Input: part model. Units: mm. Frame: model coordinates. A direction names the side the tool comes from. Give positions to 0.01 mm unless a question says otherwise; leave off trailing zeros. Loops run counter-clockwise (first coordinate to the right, second up) from the corner with the lowest first, then second, coordinate; pieces in that order, holes last. Notation, with made-up numbers: M -13,-38 L 15,-38 A17 cw 15,-32 Z; hole C 46,10.25 d7. An arc over 180 degrees is marked long. Answer as a JSON object with one key per item and string values. Group by question number.
1) Access query for faces 1 (the cylindrical face through (-2, 12.6, 0)), 2 (the cylindrical face through (-4, 7.7, -0.1)). Directions: +Z, -Z, +X, -X, +Y, -Y. A direction counts if a zero-diameter tool reaches every point of the face in a straight line with its end or side. Return the directions, or none.
2) Section query A-A on x = 2.5. Return loops of the section in (y, z).
3) First-contact query: P1, Ø8, axis at y = 4.5, z = 6, coming from the +X side; P2, Ø0.6, axis at x = 1, z = -6.5, coming from the +Y side; P3, Ø10, axis at x = -4, z = -3.5, coming from the -Y side. Flat tips, straight axial feed; report the tip coordinate or a pass-through.
4) Section query D-D on z = 8.75. Return loops of the section in (x, y).
5) Section query B-B on y = 6.5. Return loops of the section in (x, z), plus the area to 3 significant figures.
6) Ray query, L1, parallel to X at y = 5.75, z = 7.5; L2, parallel to Y at x = -1, z = 3.5; L3, parallel to Y at x = 0.5, z = 4. Return the intervals inside material, ascending.
7) Section query C-C on z = -1. Return loops of the section in (x, y), plus the area to 3 significant figures.
from build123d import *

# Parameters (mm, degrees)
F2_DEPTH      = 25.4
F2_DEPTH_BACK = 25.4
F3_DEPTH      = 25.4
F3_DEPTH_BACK = 25.4


with BuildPart() as f1:
    # F0 (on Top) → F1 (revolve)
    with BuildSketch(Plane.XY):
        with BuildLine():
            ThreePointArc((1.4741766444, 15.6340406001), (1.7521250826, 17.6942663006), (0, 18.8131241852))
            Line((0, 18.8131241852), (0, 18.009214877))
            ThreePointArc((0, 18.009214877), (0.7972124014, 17.6789986882), (1.1274285902, 16.8817862868))
            ThreePointArc((1.1274285902, 16.8817862868), (0.7972124014, 16.0845738854), (0, 15.7543576967))
            Line((0, 15.7543576967), (0, 12.7899108205))
            Line((0, 12.7899108205), (2, 12.7899108205))
            Line((2, 12.7899108205), (2, 11.7899108205))
            Line((2, 11.7899108205), (0, 11.7899108205))
            Line((0, 11.7899108205), (0, 8.4259435534))
            ThreePointArc((0, 8.4259435534), (5, 3.4259435534), (0, -1.5740564466))
            Line((0, -1.5740564466), (0, -4.8317939343))
            ThreePointArc((0, -4.8317939343), (10.2594295647, 4.7152185858), (1.4741766444, 15.6340406001))
        make_face()
    revolve(axis=Axis((0, 32.3345517981, 0), (0, -1, 0)))

    # F0 (on Top) → F2 (cut, two sides)
    with BuildSketch(Plane.XY) as f2_sk:
        with BuildLine():
            Line((2, 12.7899108205), (0, 12.7899108205))
            ThreePointArc((0, 12.7899108205), (-5, 7.7899108205), (0, 2.7899108205))
            Line((0, 2.7899108205), (2, 2.7899108205))
            Line((2, 2.7899108205), (2, 3.7899108205))
            Line((2, 3.7899108205), (0, 3.7899108205))
            ThreePointArc((0, 3.7899108205), (-4, 7.7899108205), (0, 11.7899108205))
            Line((0, 11.7899108205), (2, 11.7899108205))
            Line((2, 11.7899108205), (2, 12.7899108205))
        make_face()
        with BuildLine():
            Line((-2, -1.5740564466), (0, -1.5740564466))
            ThreePointArc((0, -1.5740564466), (5, 3.4259435534), (0, 8.4259435534))
            Line((0, 8.4259435534), (-2, 8.4259435534))
            Line((-2, 8.4259435534), (-2, 7.4259435534))
            Line((-2, 7.4259435534), (0, 7.4259435534))
            ThreePointArc((0, 7.4259435534), (4, 3.4259435534), (0, -0.5740564466))
            Line((0, -0.5740564466), (-2, -0.5740564466))
            Line((-2, -0.5740564466), (-2, -1.5740564466))
        make_face()
    extrude(amount=-F2_DEPTH, mode=Mode.SUBTRACT)
    extrude(f2_sk.sketch, amount=F2_DEPTH_BACK, mode=Mode.SUBTRACT)

    # F0 (on Top) → F3 (cut, two sides)
    with BuildSketch(Plane.XY) as f3_sk:
        with BuildLine():
            Line((0, 15.7543576967), (0, 18.009214877))
            ThreePointArc((0, 18.009214877), (-1.1274285902, 16.8817862868), (0, 15.7543576967))
        make_face()
        with BuildLine():
            ThreePointArc((1.1274285902, 16.8817862868), (0.7972124014, 17.6789986882), (0, 18.009214877))
            Line((0, 18.009214877), (0, 15.7543576967))
            ThreePointArc((0, 15.7543576967), (0.7972124014, 16.0845738854), (1.1274285902, 16.8817862868))
        make_face()
    extrude(amount=-F3_DEPTH, mode=Mode.SUBTRACT)
    extrude(f3_sk.sketch, amount=F3_DEPTH_BACK, mode=Mode.SUBTRACT)


solid = f1.part
Output:
{
 "1": {"face 1": "none", "face 2": "+Z, -Z"},
 "2": {"outline": "M -0.9,-7.69 L -0.9,7.69 A9.98 ccw Z; M 0.3,-8.55 A9.98 ccw 6.55,-9.92 L 6.55,-3 A4.33 cw 0.3,-3 Z; M 0.3,3 A4.33 cw 6.55,3 L 6.55,9.92 A9.98 ccw 0.3,8.55 Z; M 7.76,-9.71 A9.98 ccw 7.76,9.71 Z"},
 "3": {"P1": "stops at x = 10.07", "P2": "stops at y = 13.6", "P3": "stops at y = -4.83"},
 "4": {"outline": "M -4.99,7.53 A5.41 ccw 3.31,1.18 A4 ccw 0,7.43 L -2,7.43 L -2,8.43 L 0,8.43 A5 cw 5,3.39 A5.41 ccw -3.64,9.46 A4 ccw 0,3.79 L 2,3.79 L 2,2.79 L 0,2.79 A5 cw Z"},
 "5": {"outline": "M -4.83,-9.02 L -4.83,9.02 A10.23 ccw Z; M -3.79,-9.51 A10.23 ccw 2.56,-9.91 L 2.56,-3 A3.94 cw -3.79,-1.1 Z; M -3.79,1.1 A3.94 cw 2.56,3 L 2.56,9.91 A10.23 ccw -3.79,9.51 Z; M 3.94,-9.44 A10.23 ccw 3.94,9.44 Z", "area": "240 mm^2"},
 "6": {"L1": "x = -7.03 to -4.56, -3.44 to 3.26, 4.43 to 7.03", "L2": "y = -4.17 to -1.57, -0.57 to 0, 6.85 to 7.43, 8.43 to 11.66, 12.69 to 15.07", "L3": "y = -4.01 to -1.55, -0.54 to 0.47, 6.38 to 7.39, 8.4 to 11.79, 12.79 to 14.92"},
 "7": {"outline": "M -1.08,15.63 A10.24 ccw long 1.08,15.63 A1.65 ccw long Z; hole M -4.44,5.49 A4.9 ccw -2,-1.05 L -2,-1.57 L 0,-1.57 A5 ccw 0,8.43 L -2,8.43 L -2,7.9 A4.9 ccw -3.79,6.52 A4 cw 0,11.79 L 2,11.79 L 2,12.79 L -1.73,12.79 L -1.73,12.48 A5 ccw Z; hole C 0,16.88 d2.25", "area": "244 mm^2"}
}
